Source: CAD feature listing. Evaluate the final solid. Frame: model axes, mm. A direction names the side the tool comes from. Coordinates: 2 decimals unless noted, no trailing zeros. Order: outer loops, then holes, each group sorted by start corner. A loop starts at its lowest first (then second) coordinate and runs counter-clockwise, first axis right, second up. Notation, with made-up numbers: (16.5, 73) -> (43.5, 73) arc R21 ccw to (43.5, 111) -> close; hole circle Ø5 at (89.5, 25.25). An arc over 180 degrees is marked (long way). Write item = value, one per line. Start each with the question number.
Item 1: Section query C-C (y = 24.5). Output: boundary loops of the cut face in (x, z), then the cut area to 3 significant figures.
Item 2: Section query A-A (z = 5). Output: boundary loops of the cut face in (x, y), then the cut area to 3 significant figures.
Item 3: Contact query for flat-ended pins moving along their axis: pin 1 (0.8 mm diameter, centred on x = -13.5, z = 4.5, fed in from +Y); pin 2 (5 mm diameter, centred on x = -17.83, z = 5, fed in from +Y); pin 3 (4 mm diameter, centred on x = -46.5, z = 7, fed in from -Y). Output: stop coordinate, or through.
Item 4: Section query D-D (x = -28). Output: boundary loops of the cut face in (y, z), then the cut area to 3 significant figures.
Item 5: Mould query, pull axis X, two halves, no side actions, for faces 1 (the flat face through (-67, 23.574, 5)), 2 (the flat face through (-69.334, 17, 5)), 3 (the cylindrical face through (-16.93, 21.18, 7.86)). Classes: released by +X, released by -X, zero draft, split by the parting line, or undercut.
Item 6: Section query B-B (y = 19.5). Output: boundary loops of the cut face in (x, z), then the cut area to 3 significant figures.
Item 7: Ray query, line 1 along X through (y, z) = (18, 5); line 2 along X through (y, z) = (10.75, 5); line 3 along X through (y, z) = (23.5, 6.5). Return the intervals inside material, ascending. Write a range as [from, to].
Item 8: Set-up query: faces 4 (the flat face through (-40, 23, 10)), 5 (the flat face through (-19.1, 13.574, 6.3)), 6 (the flat face through (-67, 26, 6.25)), 7 (the cylindrical face through (-23.26, 27.26, 8.15)). Return all of +Z, -Z, +X, -X, +Y, -Y with unobstructed straight access to the full face (end or side cutting, diameter ignored); none if empty.
```python
from build123d import *

# Parameters (mm, degrees)
EXTRUDE_1_DEPTH     = 10
SKETCH_2_R          = 1.6
CUT_EXTRUDE_1_DEPTH = 27
SKETCH_3_R          = 3
CUT_EXTRUDE_2_DEPTH = 15
SKETCH_4_W          = 58
SKETCH_4_H          = 2.5
CUT_EXTRUDE_4_DEPTH = 5
SKETCH_5_R          = 2
CUT_EXTRUDE_5_DEPTH = 5


with BuildPart() as part:
    # 草图1 → 凸台-拉伸1 (new body)
    with BuildSketch(Plane.XY):
        with BuildLine():
            Line((-69.33427814, 6.574466706), (-69.33427814, 28.574466706))
            Line((-69.33427814, 28.574466706), (-11.33427814, 28.574466706))
            Line((-11.33427814, 28.574466706), (-11.33427814, 6.574466706))
            Line((-11.33427814, 6.574466706), (-24.33427814, 6.574466706))
            ThreePointArc((-24.33427814, 6.574466706), (-40.33427814, 22.574466706), (-56.33427814, 6.574466706))
            Line((-56.33427814, 6.574466706), (-69.33427814, 6.574466706))
        make_face()
    extrude(amount=EXTRUDE_1_DEPTH)

    # 草图2 → 切除-拉伸1 (cut)
    with BuildSketch(Plane.XZ.offset(-6.574466706)):
        with Locations(Location((-62.83427814, 5, 0), (0, 0, 270))):
            Circle(SKETCH_2_R)
        with Locations(Location((-17.83427814, 5, 0), (0, 0, 270))):
            Circle(SKETCH_2_R)
    extrude(amount=-CUT_EXTRUDE_1_DEPTH, mode=Mode.SUBTRACT)

    # 草图3 → 切除-拉伸2 (cut)
    with BuildSketch(Plane(origin=(0, 28.574466706, 0), x_dir=(1, 0, 0), z_dir=(0, 1, 0))):
        with Locations(Location((-62.83427814, -5, 0), (0, 0, 270))):
            Circle(SKETCH_3_R)
        with Locations(Location((-17.83427814, -5, 0), (0, 0, 270))):
            Circle(SKETCH_3_R)
    extrude(amount=-CUT_EXTRUDE_2_DEPTH, mode=Mode.SUBTRACT)

    # 草图4 → 切除-拉伸4 (cut)
    with BuildSketch(Plane(origin=(0, 28.574466706, 0), x_dir=(1, 0, 0), z_dir=(0, 1, 0))):
        with Locations((-40.33427814, -5)):
            Rectangle(SKETCH_4_W, SKETCH_4_H)
    extrude(amount=-CUT_EXTRUDE_4_DEPTH, mode=Mode.SUBTRACT)

    # 草图5 → 切除-拉伸5 (cut)
    with BuildSketch(Plane.XY.offset(10)):
        with Locations((-56.33427814, 25.574466706)):
            Circle(SKETCH_5_R)
        with Locations((-24.33427814, 25.574466706)):
            Circle(SKETCH_5_R)
    extrude(amount=-CUT_EXTRUDE_5_DEPTH, mode=Mode.SUBTRACT)


solid = part.part
```
Computed:
q1.outline = (-69.33, 0) -> (-11.33, 0) -> (-11.33, 3.75) -> (-15.11, 3.75) arc R3 cw to (-20.56, 3.75) -> (-60.11, 3.75) arc R3 cw to (-65.56, 3.75) -> (-69.33, 3.75) -> close; (-69.33, 6.25) -> (-65.56, 6.25) arc R3 cw to (-60.11, 6.25) -> (-58.02, 6.25) -> (-58.02, 10) -> (-69.33, 10) -> close; (-54.65, 6.25) -> (-26.02, 6.25) -> (-26.02, 10) -> (-54.65, 10) -> close; (-22.65, 6.25) -> (-20.56, 6.25) arc R3 cw to (-15.11, 6.25) -> (-11.33, 6.25) -> (-11.33, 10) -> (-22.65, 10) -> close
q1.area = 382 mm^2
q2.outline = (-69.33, 6.57) -> (-64.43, 6.57) -> (-64.43, 13.57) -> (-65.83, 13.57) -> (-65.83, 23.57) -> (-69.33, 23.57) -> close; (-61.23, 6.57) -> (-56.33, 6.57) arc R16 cw to (-24.33, 6.57) -> (-19.43, 6.57) -> (-19.43, 13.57) -> (-20.83, 13.57) -> (-20.83, 23.57) -> (-59.83, 23.57) -> (-59.83, 13.57) -> (-61.23, 13.57) -> close; (-16.23, 6.57) -> (-11.33, 6.57) -> (-11.33, 23.57) -> (-14.83, 23.57) -> (-14.83, 13.57) -> (-16.23, 13.57) -> close
q2.area = 419 mm^2
q3.pin_1 = 23.57
q3.pin_2 = 13.57
q3.pin_3 = 20.33
q4.outline = (16.77, 0) -> (28.57, 0) -> (28.57, 3.75) -> (23.57, 3.75) -> (23.57, 6.25) -> (28.57, 6.25) -> (28.57, 10) -> (16.77, 10) -> close
q4.area = 106 mm^2
q5.face_1 = zero draft
q5.face_2 = released by -X
q5.face_3 = undercut
q6.outline = (-69.33, 0) -> (-49.76, 0) -> (-49.76, 10) -> (-69.33, 10) -> close; (-30.9, 0) -> (-11.33, 0) -> (-11.33, 10) -> (-30.9, 10) -> close; hole circle Ø6 at (-62.83, 5); hole circle Ø6 at (-17.83, 5)
q6.area = 335 mm^2
q7.line_1 = [-69.33, -65.83], [-59.83, -51.54], [-29.13, -20.83], [-14.83, -11.33]
q7.line_2 = [-69.33, -64.43], [-61.23, -55.78], [-24.89, -19.43], [-16.23, -11.33]
q7.line_3 = [-69.33, -65.43], [-60.24, -20.43], [-15.24, -11.33]
q8.face_4 = +Z, +X, -X, +Y, -Y
q8.face_5 = +Y
q8.face_6 = +X, -X, +Y
q8.face_7 = +Z
